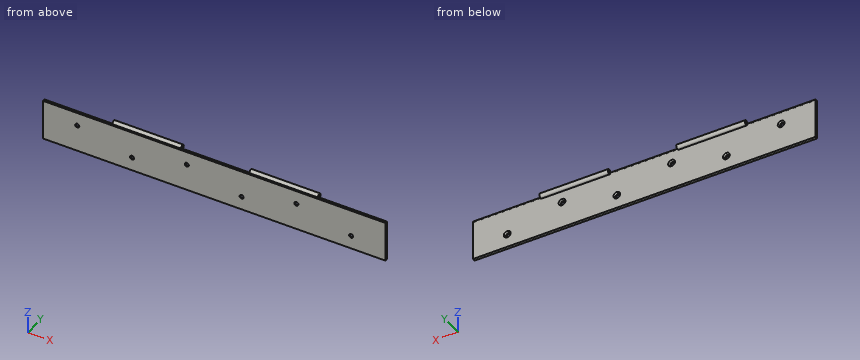
Autodesk Inventor part; units mm, degrees
ref_plane "YZ Plane" through (0, 0, 0) normal (1, 0, 0) x (0, 1, 0)
ref_plane "XZ Plane" through (0, 0, 0) normal (0, 1, 0) x (-1, 0, 0)
ref_plane "XY Plane" through (0, 0, 0) normal (0, 0, 1) x (1, 0, 0)
sketch "Sketch1" plane through (0, 0, 0) normal (0, 1, 0) x (-1, 0, 0)
  line L0 (0, 0) -> (-250, 0)
  line L1 (-250, 0) -> (-250, -30)
  line L2 (-250, -30) -> (0, -30)
  line L3 (0, -30) -> (0, 0)
  dimension "d0" = 250
  dimension "d1" = 30
extrude "Extrusion1" add sketch "Sketch1" along normal blind 2
sketch "Sketch2" plane through (250, 0, 0) normal (1, 0, 0) x (0, 0, -1)
  circle A0 centre (0, 3) radius 1.25
  circle A1 centre (0, 3) radius 1.75
  point P0 (0, 0)
  dimension "d4" = 2.5
  dimension "d5" = 3
  dimension "d6" = 3.5
extrude "Extrusion2" add sketch "Sketch2" against normal blind 250
extrude "Extrusion3" cut sketch "Sketch2" against normal blind 250 contours A0
sketch "Sketch3" plane through (250, 0, -30) normal (0, 0, -1) x (-1, 0, 0)
  line L0 (0, 2) -> (250, 2)
  line L1 (0, 2) -> (50, 2)
  line L2 (50, 2) -> (50, 4.75)
  line L3 (50, 4.75) -> (0, 4.75)
  line L4 (0, 4.75) -> (0, 2)
  line L5 (100, 4.75) -> (150, 4.75)
  line L6 (150, 4.75) -> (150, 2)
  line L7 (150, 2) -> (100, 2)
  line L8 (100, 2) -> (100, 4.75)
  line L9 (200, 4.75) -> (250, 4.75)
  line L10 (250, 4.75) -> (250, 2)
  line L11 (250, 2) -> (200, 2)
  line L12 (200, 2) -> (200, 4.75)
  point P0 (250, 0)
  point P1 (125, 2)
  point P2 (125, 2)
  point P3 (225, 2)
  dimension "d11" = 50
  dimension "d12" = 2.75
  dimension "d13" = 50
  dimension "d14" = 2.75
  dimension "d15" = 50
  dimension "d16" = 50
  dimension "d17" = 2.75
  dimension "d18" = 50
extrude "Extrusion4" cut sketch "Sketch3" against normal through all
sketch "Sketch4" plane through (200, 2, 1.4361) normal (0, 1, 0) x (1, 0, 0)
  line L0 (-200, 1.4361) -> (-200, 0)
  line L1 (-150, 0) -> (-200, 0)
  line L2 (-200, 1.4361) -> (-150, 1.4361)
  line L3 (-150, 1.4361) -> (-150, 0)
  line L4 (-150, 0) -> (-200, 0)
  line L5 (-200, 0) -> (-200, 1.4361)
  line L6 (-100, 0.1861) -> (-100, 2.6861)
  line L7 (-50, 0.6861) -> (-50, 0)
  line L8 (-100, 1.4361) -> (-50, 1.4361)
  line L9 (-50, 1.4361) -> (-50, 0)
  line L10 (-50, 0) -> (-100, 0)
  line L11 (-100, 0) -> (-100, 1.4361)
  line L12 (50, 2.1861) -> (50, 0.6861)
  line L13 (50, 0) -> (0, 0)
  line L14 (50, 1.4361) -> (0, 1.4361)
  line L15 (0, 1.4361) -> (0, 0)
  line L16 (0, 0) -> (50, 0)
  line L17 (50, 0) -> (50, 1.4361)
  point P0 (-100, 2.1861)
  point P1 (-100, 0.6861)
extrude "Extrusion5" cut sketch "Sketch4" against normal through all
sketch "Sketch5" plane through (0, 2, 0) normal (0, 1, 0) x (1, 0, 0)
  line L0 (100, 1.75) -> (100, -1.75)
  line L1 (0, 0) -> (50, 0)
  point P0 (25, 10)
  point P1 (65, 20)
  point P2 (105, 10)
  point P3 (145, 20)
  point P4 (185, 10)
  point P5 (225, 20)
  point P6 (100, 0)
  point P7 (100, 1.4361)
  dimension "d23" = 40
  dimension "d24" = 5
  dimension "d25" = 40
  dimension "d26" = 40
  dimension "d27" = 40
  dimension "d28" = 40
  dimension "d29" = 10
  dimension "d30" = 10
hole "Hole1" at (25, 2, -10) at (65, 2, -20) at (105, 2, -10) at (145, 2, -20) at (185, 2, -10) at (225, 2, -20) direction (0, -1, 0) diameter 3 end through all countersink diameter 5 countersink angle 90
equation "\"d13\" = d11"
equation "\"d15\" = d11"
equation "\"d16\" = d11"
equation "\"d18\" = d11"
properties part number "Hinge 1 of 2" material "Steel"
Can you work these out from the model? Positions are in its coordinate system, mm. Coordinates: 2 decimals unless noted, no trailing zeros. Loops run counter-clockwise (first coordinate to the right, second up) from the corner with the lowest first, then second, coordinate; pieces in that order, holes last. Notation, with made-up numbers: M -14,-9.5 L 28,-9.5 A23 ccw 28,13.5 Z; hole C 37.5,-23.5 d4. An arc over 180 degrees is marked long. Return JSON: item names as keys, results as strings. Group by question number.
Item 1: I'm going to push flat-ended pins straight in: pin 1 Ø8 at (x, z) = (185.5, -25) entering from +Y; pin 2 Ø3.5 at (x, z) = (105, -10) entering from +Y; pin 3 Ø1.8 at (x, z) = (65, -20) entering from +Y (3 decimals); pin 4 Ø1.9 at (x, y) = (88.5, 1) entering from +Z. Where does each tip first touch, or does it pass through?
Item 2: Imagine slicing it at D-D (z = -4). Please give me the cut outline in (x, y), and give its area (3 significant figures).
Item 3: If I drill on L1, parallel to Z at x = 225, y = 0.4; L2, parallel to X at y = 0.3, z = -20; L3, parallel to Z at x = 105, y = 0.25, over which ranges is the centre line in solid material (lowest first)? Write a range as from..to.
Item 4: Imagine slicing it at B-B (x = 208.5). Please give me the cut outline in (y, z).
Item 5: Imagine slicing it at C-C (x = 78.5). Please give me the cut outline in (y, z).
Item 6: Imagine slicing it at A-A (y = 3). Please give me the cut outline in (x, z).
Verdict:
{
 "1": {"pin 1": "stops at y = 2", "pin 2": "stops at y = 1.25", "pin 3": "passes through", "pin 4": "stops at z = 1.4"},
 "2": {"outline": "M 0,0 L 250,0 L 250,2 L 0,2 Z", "area": "500 mm^2"},
 "3": {"L1": "z = -30..-21.5, -18.5..0", "L2": "x = 0..63.5, 66.5..143.5, 146.5..223.5, 226.5..250", "L3": "z = -30..-11.5, -8.5..0"},
 "4": {"outline": "M 0,-30 L 2,-30 L 2,-0.75 A1.25 cw 1.75,0 L 0,0 Z"},
 "5": {"outline": "M 0,-30 L 2,-30 L 2,-1.44 A1.75 ccw long 1.25,0 L 0,0 Z; hole C 3,0 d2.5"},
 "6": {"outline": "M 50,-1.75 L 100,-1.75 L 100,-1.25 L 50,-1.25 Z; M 50,1.25 L 100,1.25 L 100,1.75 L 50,1.75 Z; M 150,-1.75 L 200,-1.75 L 200,-1.25 L 150,-1.25 Z; M 150,1.25 L 200,1.25 L 200,1.75 L 150,1.75 Z"}
}
